from build123d import *

# Parameters (mm, degrees)
CROQUIS1_R              = 1.75
CROQUIS1_R_2            = 1.05
CROQUIS1_R_3            = 1.65
CROQUIS1_R_4            = 7
CROQUIS1_W              = 24
CROQUIS1_H              = 18
CROQUIS1_W_2            = 20.5
CROQUIS1_H_2            = 9.25
CROQUIS1_W_3            = 3.8
CROQUIS1_H_3            = 2.3
CROQUIS1_W_4            = 6
CROQUIS1_H_4            = 20
CROQUIS1_W_5            = 45
CROQUIS1_H_5            = 45
SALIENTE_EXTRUIR1_DEPTH = 2


with BuildPart() as part:
    # Croquis1 → Saliente-Extruir1 (new body)
    with BuildSketch(Plane(origin=(0, 0, 0), x_dir=(1, 0, 0), z_dir=(0, 1, 0))):
        with BuildLine():
            Line((-49.462248263, -45), (80.537751737, -45))
            ThreePointArc((80.537751737, -45), (84.073285643, -43.535533906), (85.537751737, -40))
            ThreePointArc((85.537751737, -40), (79.612228902, -28.069677764), (77.037751737, -15))
            Line((77.037751737, -15), (77.037751737, 15))
            ThreePointArc((77.037751737, 15), (79.612228902, 28.069677764), (85.537751737, 40))
            ThreePointArc((85.537751737, 40), (84.073285643, 43.535533906), (80.537751737, 45))
            Line((80.537751737, 45), (-49.462248263, 45))
            ThreePointArc((-49.462248263, 45), (-63.604383887, 39.142135624), (-69.462248263, 25))
            Line((-69.462248263, 25), (-69.462248263, -25))
            ThreePointArc((-69.462248263, -25), (-63.604383887, -39.142135624), (-49.462248263, -45))
        make_face()
        with Locations(Location((-58.462248263, -14, 0), (0, 0, 270))):
            Circle(CROQUIS1_R, mode=Mode.SUBTRACT)
        with Locations(Location((-58.462248263, 14, 0), (0, 0, 90))):
            Circle(CROQUIS1_R, mode=Mode.SUBTRACT)
        with Locations(Location((71.365251737, 0, 0), (0, 0, 270))):
            Circle(CROQUIS1_R_2, mode=Mode.SUBTRACT)
        with Locations(Location((47.465251737, 0, 0), (0, 0, 270))):
            Circle(CROQUIS1_R_2, mode=Mode.SUBTRACT)
        with Locations(Location((-43.462248263, 0, 0), (0, 0, 270))):
            Circle(CROQUIS1_R_3, mode=Mode.SUBTRACT)
        with Locations(Location((12.417751737, 0, 0), (0, 0, 270))):
            Circle(CROQUIS1_R_3, mode=Mode.SUBTRACT)
        with Locations(Location((-58.462248263, 0, 0), (0, 0, 270))):
            Circle(CROQUIS1_R_4, mode=Mode.SUBTRACT)
        with Locations(Location((41.537751737, 0, 0), (0, 0, 270))):
            Circle(CROQUIS1_R_3, mode=Mode.SUBTRACT)
        with Locations(Location((17.977751737, 8, 0), (0, 0, 270))):
            Circle(CROQUIS1_R, mode=Mode.SUBTRACT)
        with Locations(Location((17.977751737, -18.7345, 0), (0, 0, 270))):
            Circle(CROQUIS1_R, mode=Mode.SUBTRACT)
        with Locations((52.037751737, -25)):
            Rectangle(CROQUIS1_W, CROQUIS1_H, mode=Mode.SUBTRACT)
        with Locations((59.415251737, 0)):
            Rectangle(CROQUIS1_W_2, CROQUIS1_H_2, mode=Mode.SUBTRACT)
        with Locations((30.037751737, 41.35)):
            Rectangle(CROQUIS1_W_3, CROQUIS1_H_3, mode=Mode.SUBTRACT)
        with Locations((76.137751737, 41.35)):
            Rectangle(CROQUIS1_W_3, CROQUIS1_H_3, mode=Mode.SUBTRACT)
        with Locations((76.137751737, -41.35)):
            Rectangle(CROQUIS1_W_3, CROQUIS1_H_3, mode=Mode.SUBTRACT)
        with Locations((30.037751737, -41.35)):
            Rectangle(CROQUIS1_W_3, CROQUIS1_H_3, mode=Mode.SUBTRACT)
        with Locations((33.037751737, 0)):
            Rectangle(CROQUIS1_W_4, CROQUIS1_H_4, mode=Mode.SUBTRACT)
        with Locations((-15.522248263, 0)):
            Rectangle(CROQUIS1_W_5, CROQUIS1_H_5, mode=Mode.SUBTRACT)
        with Locations((52.037751737, 25)):
            Rectangle(CROQUIS1_W, CROQUIS1_H, mode=Mode.SUBTRACT)
    extrude(amount=SALIENTE_EXTRUIR1_DEPTH)


solid = part.part
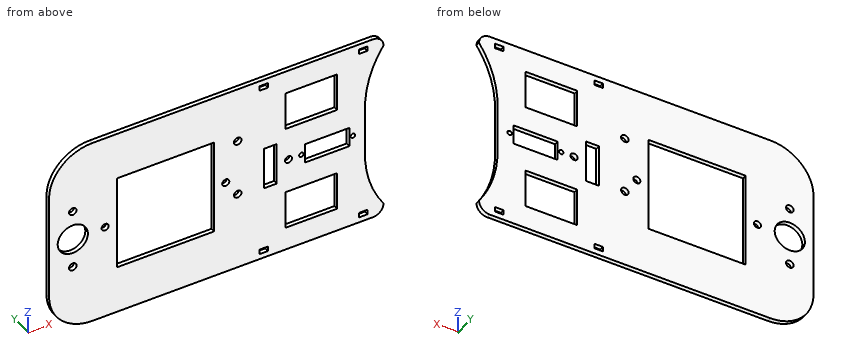
Input: part model. Units: mm. Frame: model coordinates. Coordinates: 2 decimals unless noted, no trailing zeros. Loops run counter-clockwise (first coordinate to the right, second up) from the corner with the lowest first, then second, coordinate; pieces in that order, holes last. Notation, with made-up numbers: (0.25, -33.75) -> (59.25, -33.75) arc R32 ccw to (59.25, -2.75) -> close; hole circle Ø10 at (71, 39). An arc over 180 degrees is marked (long way). Write item = value, one per line. Start each with the question number.
Item 1: Cut plane D-D, the plane z = -37. Return loops of the section in (x, y).
Item 2: Cut plane C-C, the plane y = 0.45. Count the separate pieces of the cut face and the enclosed holes in it, plus the area to 3 significant figures.
Item 3: Cut plane B-B, the plane x = 4. Return loops of the section in (y, z), plus the area to 3 significant figures.
Item 4: Cut plane A-A, the plane x = 59. Return loops of the section in (y, z) (3 decimals), plus the area to 3 significant figures.
Item 5: First-contact query: P1, Ø1.3, axis at x = 47.47, z = 0, coming from the -Y side; P2, Ø0.6, axis at y = 1.5, z = 25.5, coming from the +X side; P3, Ø5, axis at x = -11.5, z = -22, coming from the +Y side; P4, Ø0.6, axis at y = 1.5, z = -28.5, coming from the -X side. Flat tips, straight axial feed; report the tip coordinate or a pass-through.
Item 6: Material intervals for line 1 (X direction, y = 1.4, z = -8); line 2 (Z direction, x = -18, y = 0.1); line 3 (X direction, y = 0.5, z = -13), sorted ascending.
Ans:
q1.outline = (-65.46, 0) -> (83.66, 0) -> (83.66, 2) -> (-65.46, 2) -> close
q2.separate_pieces = 1
q2.enclosed_holes = 19
q2.area = 9,780 mm²
q3.outline = (0, -45) -> (2, -45) -> (2, -22.5) -> (0, -22.5) -> close; (0, 22.5) -> (2, 22.5) -> (2, 45) -> (0, 45) -> close
q3.area = 90.0 mm²
q4.outline = (0, -45) -> (2, -45) -> (2, -34) -> (0, -34) -> close; (0, -16) -> (2, -16) -> (2, -4.625) -> (0, -4.625) -> close; (0, 4.625) -> (2, 4.625) -> (2, 16) -> (0, 16) -> close; (0, 34) -> (2, 34) -> (2, 45) -> (0, 45) -> close
q4.area = 89.5 mm²
q5.P1 = through
q5.P2 = 78.9
q5.P3 = 2
q5.P4 = -69.2
q6.line_1 = -69.46 to -38.02, 6.98 to 16.23, 19.73 to 30.04, 36.04 to 77.04
q6.line_2 = -45 to -22.5, 22.5 to 45
q6.line_3 = -69.46 to -59.9, -57.03 to -38.02, 6.98 to 77.04
